```python
from build123d import *

# Parameters (mm, degrees)
EXTRUDE_2_DEPTH     = 5
EXTRUDE_2_2_DEPTH   = 5
EXTRUDE_3_DEPTH     = 50
EXTRUDE_4_DEPTH     = 10
CUT_EXTRUDE_1_DEPTH = 7.5
SKETCH_9_R          = 1.25
CUT_EXTRUDE_3_DEPTH = 20
SKETCH_10_R         = 8
SKETCH_10_R_2       = 1.25
CUT_EXTRUDE_7_DEPTH = 5
SKETCH_1_9_R        = 1.25
EXTRUDE_5_DEPTH     = 45
SKETCH_14_R         = 1.25
CUT_EXTRUDE_8_DEPTH = 14
EXTRUDE_6_DEPTH     = 15


# Read off the part's stored shape, not the designer's step: the extrude step
with BuildPart() as part:
    # Sketch 1 → Extrude 2 (new body)
    with BuildSketch(Plane(origin=(0, 0, 0), x_dir=(1, 0, 0), z_dir=(0, 1, 0))):
        with BuildLine():
            Line((6.548408352, 75.246242124), (-83.374180902, 75.246242124))
            Line((-83.374180902, 75.246242124), (-83.374180902, 65.246242124))
            ThreePointArc((-83.374180902, 65.246242124), (-84.838646996, 61.710708218), (-88.374180902, 60.246242124))
            Line((-88.374180902, 60.246242124), (-98.374180902, 60.246242124))
            Line((-98.374180902, 60.246242124), (-98.374180902, -54.753757876))
            Line((-98.374180902, -54.753757876), (-88.374180902, -54.753757876))
            ThreePointArc((-88.374180902, -54.753757876), (-84.838646996, -56.21822397), (-83.374180902, -59.753757876))
            Line((-83.374180902, -59.753757876), (-83.374180902, -69.753757876))
            Line((-83.374180902, -69.753757876), (46.625819098, -69.753757876))
            Line((46.625819098, -69.753757876), (46.625819098, -59.753757876))
            ThreePointArc((46.625819098, -59.753757876), (48.090285193, -56.21822397), (51.625819098, -54.753757876))
            Line((51.625819098, -54.753757876), (61.625819098, -54.753757876))
            Line((61.625819098, -54.753757876), (61.625819098, 14.619924984))
            Line((61.625819098, 14.619924984), (55.067595409, 14.619924984))
            ThreePointArc((55.067595409, 14.619924984), (50.381304866, 17.876743713), (51.799973847, 23.404452606))
            Line((51.799973847, 23.404452606), (56.763929588, 27.690411234))
            Line((56.763929588, 27.690411234), (21.686518841, 68.316728374))
            Line((21.686518841, 68.316728374), (14.816029914, 62.384638559))
            ThreePointArc((14.816029914, 62.384638559), (9.467315828, 61.622843062), (6.548408352, 66.169166182))
            Line((6.548408352, 66.169166182), (6.548408352, 75.246242124))
        make_face()
        Polygon((-31.470797546, 9.525154804), (-22.387931252, 17.367446554), (-2.782201877, -5.33971918), (-11.865068171, -13.18201093), align=None, mode=Mode.SUBTRACT)
    extrude(amount=EXTRUDE_2_DEPTH)

    # Sketch 1_6 → Extrude 3 (add)
    with BuildSketch(Plane(origin=(0, 0, 0), x_dir=(1, 0, 0), z_dir=(0, 1, 0))):
        with BuildLine():
            Line((66.625819098, 34.900965901), (66.625819098, -62.253757876))
            ThreePointArc((66.625819098, -62.253757876), (62.964653863, -71.092592641), (54.125819098, -74.753757876))
            Line((54.125819098, -74.753757876), (-90.874180902, -74.753757876))
            ThreePointArc((-90.874180902, -74.753757876), (-99.713015666, -71.092592641), (-103.374180902, -62.253757876))
            Line((-103.374180902, -62.253757876), (-103.374180902, 67.746242124))
            ThreePointArc((-103.374180902, 67.746242124), (-99.713015666, 76.585076889), (-90.874180902, 80.246242124))
            Line((-90.874180902, 80.246242124), (26.449603474, 80.246242124))
            ThreePointArc((26.449603474, 80.246242124), (29.57124226, 79.565726803), (32.126394907, 77.647674468))
            Line((32.126394907, 77.647674468), (64.802610532, 39.802398244))
            ThreePointArc((64.802610532, 39.802398244), (66.155254913, 37.515737807), (66.625819098, 34.900965901))
        make_face()
        with BuildLine():
            ThreePointArc((61.625819098, 19.269608073), (61.155254913, 21.88437998), (59.802610532, 24.171040417))
            Line((59.802610532, 24.171040417), (17.947110848, 72.647674468))
            ThreePointArc((17.947110848, 72.647674468), (15.3919582, 74.565726803), (12.270319414, 75.246242124))
            Line((12.270319414, 75.246242124), (-90.874180902, 75.246242124))
            ThreePointArc((-90.874180902, 75.246242124), (-96.17748176, 73.049542983), (-98.374180902, 67.746242124))
            Line((-98.374180902, 67.746242124), (-98.374180902, -62.253757876))
            ThreePointArc((-98.374180902, -62.253757876), (-96.17748176, -67.557058735), (-90.874180902, -69.753757876))
            Line((-90.874180902, -69.753757876), (54.125819098, -69.753757876))
            ThreePointArc((54.125819098, -69.753757876), (59.429119957, -67.557058735), (61.625819098, -62.253757876))
            Line((61.625819098, -62.253757876), (61.625819098, 19.269608073))
        make_face(mode=Mode.SUBTRACT)
    extrude(amount=EXTRUDE_3_DEPTH)

    # Extrude 4 outline → Extrude 4 (add)
    with BuildSketch(Plane(origin=(0, 0, 0), x_dir=(1, 0, 0), z_dir=(0, 1, 0))):
        Polygon((-6.5667295, -8.607340743), (-26.172458875, 14.099824991), (-27.686269924, 12.792776366), (-8.080540549, -9.914389368), align=None)
    extrude(amount=EXTRUDE_4_DEPTH)

    # Sketch 6 → Cut-Extrude 1 (cut)
    with BuildSketch(Plane(origin=(56.814304212, 0, -49.054377198), x_dir=(-0.6535243124977221, 0, -0.7569055244707755), z_dir=(0.7569055244707754, 0, -0.653524312497722))):
        with BuildLine():
            Line((9.676573622, 24.2), (9.676573622, 21.9))
            Line((9.676573622, 21.9), (15.876573622, 21.9))
            Line((15.876573622, 21.9), (15.876573622, 24.2))
            ThreePointArc((15.876573622, 24.2), (16.676573622, 25), (15.876573622, 25.8))
            Line((15.876573622, 25.8), (15.876573622, 27.1))
            Line((15.876573622, 27.1), (14.876573622, 28.1))
            Line((14.876573622, 28.1), (10.676573622, 28.1))
            Line((10.676573622, 28.1), (9.676573622, 27.1))
            Line((9.676573622, 27.1), (9.676573622, 25.8))
            ThreePointArc((9.676573622, 25.8), (8.876573622, 25), (9.676573622, 24.2))
        make_face()
    extrude(amount=-CUT_EXTRUDE_1_DEPTH, mode=Mode.SUBTRACT)

    # Sketch 9 → Cut-Extrude 3 (cut)
    with BuildSketch(Plane(origin=(51.137512779, 0, -44.152944854), x_dir=(-0.6535243124977224, 0, -0.7569055244707754), z_dir=(0.7569055244707754, 0, -0.6535243124977224))):
        with Locations((12.776573622, 25)):
            Circle(SKETCH_9_R)
    extrude(amount=-CUT_EXTRUDE_3_DEPTH, mode=Mode.SUBTRACT)

    # Sketch 10 → Cut-Extrude 7 (cut)
    with BuildSketch(Plane.ZY.offset(103.374180902)):
        with Locations((-2.746242124, 25)):
            Circle(SKETCH_10_R)
        with Locations((-59.046242124, 24)):
            Circle(SKETCH_10_R_2)
        with Locations((53.553757876, 24)):
            Circle(SKETCH_10_R_2)
    extrude(amount=-CUT_EXTRUDE_7_DEPTH, mode=Mode.SUBTRACT)

    # Sketch 1_9 → Extrude 5 (add)
    # profile 1 of 5: a face of its own
    with BuildSketch(Plane(origin=(0, 0, 0), x_dir=(1, 0, 0), z_dir=(0, 1, 0))):
        with BuildLine():
            Line((-83.374180902, 75.246242124), (-90.874180902, 75.246242124))
            ThreePointArc((-90.874180902, 75.246242124), (-96.17748176, 73.049542983), (-98.374180902, 67.746242124))
            Line((-98.374180902, 67.746242124), (-98.374180902, 60.246242124))
            Line((-98.374180902, 60.246242124), (-88.374180902, 60.246242124))
            ThreePointArc((-88.374180902, 60.246242124), (-84.838646996, 61.710708218), (-83.374180902, 65.246242124))
            Line((-83.374180902, 65.246242124), (-83.374180902, 75.246242124))
        make_face()
        with Locations(Location((-90.874180902, 67.746242124, 0), (0, 0, 90))):
            Circle(SKETCH_1_9_R, mode=Mode.SUBTRACT)
    # profile 2 of 5: a face of its own
    with BuildSketch(Plane(origin=(0, 0, 0), x_dir=(1, 0, 0), z_dir=(0, 1, 0))):
        with BuildLine():
            Line((-88.374180902, -54.753757876), (-98.374180902, -54.753757876))
            Line((-98.374180902, -54.753757876), (-98.374180902, -62.253757876))
            ThreePointArc((-98.374180902, -62.253757876), (-96.17748176, -67.557058735), (-90.874180902, -69.753757876))
            Line((-90.874180902, -69.753757876), (-83.374180902, -69.753757876))
            Line((-83.374180902, -69.753757876), (-83.374180902, -59.753757876))
            ThreePointArc((-83.374180902, -59.753757876), (-84.838646996, -56.21822397), (-88.374180902, -54.753757876))
        make_face()
        with Locations(Location((-90.874180902, -62.253757876, 0), (0, 0, 90))):
            Circle(SKETCH_1_9_R, mode=Mode.SUBTRACT)
    # profile 3 of 5: a face of its own
    with BuildSketch(Plane(origin=(0, 0, 0), x_dir=(1, 0, 0), z_dir=(0, 1, 0))):
        with BuildLine():
            Line((46.625819098, -59.753757876), (46.625819098, -69.753757876))
            Line((46.625819098, -69.753757876), (54.125819098, -69.753757876))
            ThreePointArc((54.125819098, -69.753757876), (59.429119957, -67.557058735), (61.625819098, -62.253757876))
            Line((61.625819098, -62.253757876), (61.625819098, -54.753757876))
            Line((61.625819098, -54.753757876), (51.625819098, -54.753757876))
            ThreePointArc((51.625819098, -54.753757876), (48.090285193, -56.21822397), (46.625819098, -59.753757876))
        make_face()
        with Locations(Location((54.125819098, -62.253757876, 0), (0, 0, 90))):
            Circle(SKETCH_1_9_R, mode=Mode.SUBTRACT)
    # profile 4 of 5: a face of its own
    with BuildSketch(Plane(origin=(0, 0, 0), x_dir=(1, 0, 0), z_dir=(0, 1, 0))):
        with BuildLine():
            Line((59.802610532, 24.171040417), (56.763929588, 27.690411234))
            Line((56.763929588, 27.690411234), (51.799973847, 23.404452606))
            ThreePointArc((51.799973847, 23.404452606), (50.381304866, 17.876743713), (55.067595409, 14.619924984))
            Line((55.067595409, 14.619924984), (61.625819098, 14.619924984))
            Line((61.625819098, 14.619924984), (61.625819098, 19.269608073))
            ThreePointArc((61.625819098, 19.269608073), (61.155254913, 21.88437998), (59.802610532, 24.171040417))
        make_face()
        with Locations(Location((55.067595409, 19.619924984, 0), (0, 0, 90))):
            Circle(SKETCH_1_9_R, mode=Mode.SUBTRACT)
    # profile 5 of 5: a face of its own
    with BuildSketch(Plane(origin=(0, 0, 0), x_dir=(1, 0, 0), z_dir=(0, 1, 0))):
        with BuildLine():
            Line((12.270319414, 75.246242124), (6.548408352, 75.246242124))
            Line((6.548408352, 75.246242124), (6.548408352, 66.169166182))
            ThreePointArc((6.548408352, 66.169166182), (9.467315828, 61.622843062), (14.816029914, 62.384638559))
            Line((14.816029914, 62.384638559), (21.686518841, 68.316728374))
            Line((21.686518841, 68.316728374), (17.947110848, 72.647674468))
            ThreePointArc((17.947110848, 72.647674468), (15.3919582, 74.565726803), (12.270319414, 75.246242124))
        make_face()
        with Locations(Location((11.548408352, 66.169166182, 0), (0, 0, 90))):
            Circle(SKETCH_1_9_R, mode=Mode.SUBTRACT)
    extrude(amount=EXTRUDE_5_DEPTH)

    # Sketch 14 → Cut-Extrude 8 (cut)
    with BuildSketch(Plane(origin=(46.21762687, 0, -39.905036823), x_dir=(0.6535243124977226, 0, 0.7569055244707751), z_dir=(-0.7569055244707751, 0, 0.6535243124977226))):
        with Locations((2.223426378, 25)):
            Circle(SKETCH_14_R)
        with Locations((-27.776573622, 25)):
            Circle(SKETCH_14_R)
    extrude(amount=-CUT_EXTRUDE_8_DEPTH, mode=Mode.SUBTRACT)



with BuildPart() as body_2:
    # Sketch 1 → Extrude 2 2 (new body)
    with BuildSketch(Plane(origin=(0, 0, 0), x_dir=(1, 0, 0), z_dir=(0, 1, 0))):
        Polygon((-9.834351062, -4.822813121), (-22.904837312, 10.315297369), (-24.418648361, 9.008248744), (-11.348162111, -6.129861746), align=None)
    extrude(amount=EXTRUDE_2_2_DEPTH)


with BuildPart() as part_1:
    add(part.part)

    add(body_2.part)  # Extrude 6 merges body 2
    # Sketch 1_10 → Extrude 6 (add)
    with BuildSketch(Plane(origin=(0, 0, 0), x_dir=(1, 0, 0), z_dir=(0, 1, 0))):
        Polygon((-26.172458875, 14.099824991), (-22.904837312, 10.315297369), (-9.834351062, -4.822813121), (-6.5667295, -8.607340743), (-2.782201877, -5.33971918), (-22.387931252, 17.367446554), align=None)
        Polygon((-11.348162111, -6.129861746), (-24.418648361, 9.008248744), (-27.686269924, 12.792776366), (-31.470797546, 9.525154804), (-11.865068171, -13.18201093), (-8.080540549, -9.914389368), align=None)
    extrude(amount=EXTRUDE_6_DEPTH)


solid = part_1.part
```
The model under review builds one solid part; all positions refer to its coordinate system, in mm. A direction names the side the tool comes from. Give positions to 0.01 mm unless a question says otherwise; leave off trailing zeros. Write each loop counter-clockwise with the first axis right and the second up, starting at its lowest first coordinate (ties: lowest second). Pieces come first, ordered by that corner, then holes. Notation, with made-up numbers: M 88,27.5 L 120,27.5 A34 ccw 120,57.5 Z; hole C -20,83.5 d2. An arc over 180 degrees is marked long. Write item = value, one per line. Start each with the question number.
Q1. Machinability: for faces 4 (the face through (57, 25, 54.754)), 5 (the face through (46, 28.1, -56)), which of the approach directions +Z, -Z, +X, -X, +Y, -Y give a long, thin tool a straight path to every point of the face, cutting with its end or side? Answer none if there is none.
Q2. We need section A-A (z = 57.5). State the section outline as (x, y) points.
Q3. We need section C-C (z = -32.5). State the section outline as (x, y) points.
Q4. Clearance check with flat-ended pins moving along their axes: pin 1 (7 mm diameter, centred on x = -14.5, z = 3.5, fed in from +Y); pin 2 (5 mm diameter, centred on x = 56.5, y = 29, fed in from -Z); pin 3 (4 mm diameter, centred on x = -90.87, z = -67.75, fed in from +Y). State where each tip first meets the part, or that it passes through.
Q5. For line 1 (X direction, y = 46, z = -15.5); line 2 (Z direction, x = 55, y = 12); line 3 (X direction, y = 39, z = -20), list the stretches that pass through material, from the lowest coordinate up.
Q6. We need section B-B (y = 41). Give the number of separate pieces and of enclosed holes in the cut face, plus the area to 3 significant figures.
Q7. Mouldability with a two-part tool opening along X and no side actions: class faces 1 (the face through (-21.805, 9.93, 1.669)), 2 (the face through (66.626, 25, 13)), 3 (the face through (-20, 0, -4)) as released by +X, released by -X, zero draft, split by the parting line, or undercut.
Result set:
q1.face_4 = +Y
q1.face_5 = none
q2.outline = M -103.37,0 L 66.63,0 L 66.63,50 L 61.63,50 L 61.63,45 L 47.16,45 L 47.16,5 L -83.91,5 L -83.91,45 L -98.37,45 L -98.37,50 L -103.37,50 Z
q3.outline = M -103.37,0 L 66.63,0 L 66.63,50 L 52.61,50 L 52.61,5 L -98.37,5 L -98.37,50 L -103.37,50 Z
q4.pin_1 = 15
q4.pin_2 = -52.31
q4.pin_3 = 45
q5.line_1 = -103.37 to -98.37, 61.63 to 66.63
q5.line_2 = -51.16 to -29.73, -26.17 to -20.87, -18.37 to -14.62, 54.75 to 61.36, 63.15 to 74.72
q5.line_3 = -103.37 to -98.37, 50.08 to 53.88, 56.26 to 66.63
q6.separate_pieces = 1
q6.enclosed_holes = 6
q6.area = 4,390 mm2
q7.face_1 = undercut
q7.face_2 = released by +X
q7.face_3 = zero draft
